Autodesk Inventor part; units mm, degrees
ref_plane "1_XY" through (3, 0, 0) normal (1, 0, 0) x (0, 0, -1)
ref_plane "1_YZ" through (3, 0, 0) normal (0, 0, -1) x (0, 1, 0)
ref_plane "1_ZX" through (3, 0, 0) normal (0, 1, 0) x (1, 0, 0)
sketch "Sketch_3" plane through (0, 0, 0) normal (0, 0, 1) x (1, 0, 0)
  line L0 (5.7, 0) -> (0, 0)
  line L1 (0, 12.2) -> (0, 9.69)
  arc A0 (0, 9.69) -> (0.15, 9.54) centre (0.15, 9.69) ccw
  line L2 (0.15, 9.54) -> (0.605, 9.54)
  line L3 (0.605, 9.54) -> (0.605, 9.3335)
  line L4 (0.605, 9.3335) -> (2.1386, 9.3335)
  arc A1 (3.8614, 9.3335) -> (2.1386, 9.3335) centre (3, 8) ccw
  line L5 (3.8614, 9.3335) -> (5.4, 9.3335)
  line L6 (5.4, 9.3335) -> (5.4, 9.54)
  line L7 (5.4, 9.54) -> (5.85, 9.54)
  arc A2 (5.85, 9.54) -> (6, 9.69) centre (5.85, 9.69) ccw
  line L8 (6, 9.69) -> (6, 10.7)
  arc A3 (6, 10.7) -> (5.7, 11) centre (5.7, 10.7) ccw
  line L9 (5.7, 11) -> (1.5, 11)
  line L10 (1.5, 11) -> (1.5, 12.2)
  line L11 (1.5, 12.2) -> (1.2, 12.5)
  line L12 (1.2, 12.5) -> (0.3, 12.5)
  line L13 (0.3, 12.5) -> (0, 12.2)
revolve "Revolution1" add sketch "Sketch_3" angle 360 about axis through (5.7, 0, 0) along (1, 0, 0)
ref_plane "1_XY" through (3, 0, 0) normal (1, 0, 0) x (0, 0, -1)
ref_plane "1_YZ" through (3, 0, 0) normal (0, 0, -1) x (0, 1, 0)
ref_plane "1_ZX" through (3, 0, 0) normal (0, 1, 0) x (1, 0, 0)
properties part number "RF-2210X2HH_or"
Read the model definition and answer for the solid it produces. Units are mm, in the model's axes. A direction names the side the tool comes from. Round coordinates to 2 decimals unless told otherwise and drop trailing zeros. Order: outer loops, then holes, each group sorted by start corner. A loop starts at its lowest first (then second) coordinate and runs counter-clockwise, first axis right, second up.
1) The part is cut by section C-C on x = 0.9. Write down the section's boundary in (y, z), plus the area to 3 significant figures.
2) Straight lines are drawn through the part: L1, parallel to Z at x = 5.6, y = 0; L2, parallel to Z at x = 4.35, y = 6.5; L3, parallel to Y at x = 5.05, z = -0.5. For each, find the intervals that lie inside material, in ascending order.
3) Flat-ended cylindrical pins translate along their axes: pin 1 (2 mm diameter, centred on x = 4.5, z = -5, fed in from -Y); pin 2 (1.5 mm diameter, centred on x = 5.5, z = 7, fed in from -Y); pin 3 (3 mm diameter, centred on x = 1, y = 5, fed in from -Z). Find the tip coordinate at first contact, or state that the pin passes through.
4) The part is cut by section B-B on x = 4.55. Write down the section's boundary in (y, z), plus the area to 3 significant figures.
5) For faces 1 (the face through (1.5, -2, 11)), 2 (the face through (1.38, 4.31, -8.28)), 3 (the face through (0.38, -1.24, 9.46)), determine the directions among +Z, -Z, +X, -X, +Y, -Y from which every point of the face is accessible in a straight line to the end or side of a thin tool.
6) The mould has two halves that part along Y. Classify faces 4 (the face through (3.57, -2.38, 10.74)), 5 (the face through (0, 4, 9)), 6 (the face through (5.63, -1.24, 9.46)): released by +Y, released by -Y, zero draft, split by the parting line, or undercut.
Resolved:
1. outline: circle Ø25 at (0, 0); hole circle Ø18.67 at (0, 0)
1. area: 217 mm2
2. L1: z = -11 to -9.54, 9.54 to 11
2. L2: z = -8.87 to -6.7, 6.7 to 8.87
2. L3: y = -10.99 to -9.32, 9.32 to 10.99
3. pin 1: stops at y = -10.25
3. pin 2: stops at y = -9.05
3. pin 3: stops at z = -12
4. outline: circle Ø22 at (0, 0); hole circle Ø18.67 at (0, 0)
4. area: 106 mm2
5. face 1: +X
5. face 2: +X, -X
5. face 3: -X
6. face 4: split by the parting line
6. face 5: zero draft
6. face 6: undercut
